Design review of the part built by this model. Coordinates are the model's own, in mm. A direction names the side the tool comes from. Give positions to 0.01 mm unless a question says otherwise; leave off trailing zeros. Use CSV: the item, a comma, the result in double quotes.
from build123d import *

# Parameters (mm, degrees)
BOSS_EXTRUDE1_DEPTH      = 5
CUT_EXTRUDE1_DEPTH       = 1
BOSS_EXTRUDE2_DEPTH      = 0.0254
BOSS_EXTRUDE2_DEPTH_BACK = 1
SKETCH3_W                = 0.777152918
SKETCH3_H                = 1.679205413
FILLET1_R                = 0.0254


with BuildPart() as part:
    # Sketch1 → Boss-Extrude1 (new body)
    with BuildSketch(Plane(origin=(0, 0, 0), x_dir=(1, 0, 0), z_dir=(0, 1, 0))):
        Polygon((-3, 2), (-2, 3), (2, 3), (3, 2), (3, -2), (2, -3), (-2, -3), (-3, -2), align=None)
    extrude(amount=BOSS_EXTRUDE1_DEPTH)

    # Sketch2 → Cut-Extrude1 (cut)
    with BuildSketch(Plane(origin=(0, 5, 0), x_dir=(1, 0, 0), z_dir=(0, 1, 0))):
        Polygon((3, -2), (3, 2), (2, 3), (-2, 3), (-3, 2), (-3, -2), (-2, -3), (2, -3), align=None)
        Polygon((2.492, -1.78957951), (2.492, 1.78957951), (1.78957951, 2.492), (-1.78957951, 2.492), (-2.492, 1.78957951), (-2.492, -1.78957951), (-1.78957951, -2.492), (1.78957951, -2.492), align=None, mode=Mode.SUBTRACT)
    extrude(amount=-CUT_EXTRUDE1_DEPTH, mode=Mode.SUBTRACT)

    # Sketch3 → Boss-Extrude2 (add, two sides: drawn at the far end of the back side and taken through both)
    with BuildSketch(Plane.XZ.offset(-BOSS_EXTRUDE2_DEPTH_BACK)):
        with Locations((0, 2.210397294)):
            Rectangle(SKETCH3_W, SKETCH3_H)
        with Locations((0, -2.210397294)):
            Rectangle(SKETCH3_W, SKETCH3_H)
    extrude(amount=BOSS_EXTRUDE2_DEPTH + BOSS_EXTRUDE2_DEPTH_BACK)

    # Fillet1
    fillet1_edges = [part.edges().sort_by_distance(p)[0] for p in [
        (0.388576459, 0, 2.185397293),
        (0.388576459, 0, -2.185397293),
        (0, 0, -1.370794587),
        (-0.388576459, 0, -2.185397293),
        (-0.388576459, 0, 2.185397293),
        (0, 0, 1.370794587),
        (1.78957951, 4.5, -2.492),
        (2.492, 4.5, -1.78957951),
        (2.492, 4.5, 1.78957951),
        (1.78957951, 4.5, 2.492),
        (-1.78957951, 4.5, 2.492),
        (-2.492, 4.5, 1.78957951),
        (-2.492, 4.5, -1.78957951),
        (-1.78957951, 4.5, -2.492),
        (0, 5, 2.492),
        (-2.140789755, 5, 2.140789755),
        (-2.492, 5, 0),
        (-2.140789755, 5, -2.140789755),
        (0, 5, -2.492),
        (2.140789755, 5, -2.140789755),
        (2.492, 5, 0),
        (2.140789755, 5, 2.140789755),
        (2.140789755, 4, -2.140789755),
        (0, 4, -2.492),
        (-2.140789755, 4, -2.140789755),
        (-2.492, 4, 0),
        (-2.140789755, 4, 2.140789755),
        (0, 4, 2.492),
        (2.140789755, 4, 2.140789755),
        (2.492, 4, 0),
        (0, 4, -3),
        (-1.19428823, 0, -3),
        (-0.388576459, 0.5, -3),
        (0, 1, -3),
        (0.388576459, 0.5, -3),
        (1.19428823, 0, -3),
        (-2.5, 0, -2.5),
        (-2, 2, -3),
        (-2.5, 4, -2.5),
        (-3, 0, 0),
        (-3, 2, -2),
        (-3, 4, 0),
        (-2.5, 0, 2.5),
        (-3, 2, 2),
        (-2.5, 4, 2.5),
        (-2, 2, 3),
        (0, 4, 3),
        (1.19428823, 0, 3),
        (0.388576459, 0.5, 3),
        (0, 1, 3),
        (-0.388576459, 0.5, 3),
        (-1.19428823, 0, 3),
        (2.5, 0, 2.5),
        (2, 2, 3),
        (2.5, 4, 2.5),
        (3, 0, 0),
        (3, 2, 2),
        (3, 4, 0),
        (2, 2, -3),
        (2.5, 0, -2.5),
        (3, 2, -2),
        (2.5, 4, -2.5),
    ]]
    fillet(fillet1_edges, radius=FILLET1_R - 0.0001)  # a hair under: the kernel refuses the full size


solid = part.part
(1) Machinability: for faces 1 (the flat face through (0, 4.5, -2.492)), 2 (the flat face through (0, 4, -2.7)), 3 (the flat face through (2.5, 2, -2.5)), 4 (the flat face through (-2.492, 4.5, 0)), which of the approach directions +Z, -Z, +X, -X, +Y, -Y give a long, thin tool a straight path to every point of the face, cutting with its end or side? Answer none if there is none.
A:
face 1,"-Z, +X, -X, +Y"
face 2,"+Y"
face 3,"-Z, +X, +Y, -Y"
face 4,"+Z, -Z, -X, +Y"
(2) Clearance check with flat-ended pins moving along their axes: P1, Ø0.5, axis at y = 4.5, z = 0, coming from the -X side; P2, Ø2, axis at x = 1, y = 2, coming from the +Z side; P3, Ø0.8, axis at y = 4.5, z = -0.5, coming from the +X side. State where each tip first meets the part, or that it passes through.
A:
P1,"x = -2.49"
P2,"z = 3"
P3,"x = 2.49"
(3) Wall thickness on line 1 along Z through (x, y) = (1.55, 0.6); line 2 along Y through (x, z) = (-1.4, 2); line 3 along X through (y, z) = (3, -2.5): over which ranges is each line inside the solid? List them lowest first. Write a range as [from, to].
A:
line 1,"[-3, 3]"
line 2,"[0, 5]"
line 3,"[-2.5, 2.5]"
